Geometry: final body of the model. Coordinates: model frame, mm. A direction names the side the tool comes from. Give positions to 0.01 mm unless a question says otherwise; leave off trailing zeros. Write each loop counter-clockwise with the first axis right and the second up, starting at its lowest first coordinate (ties: lowest second). Pieces come first, ordered by that corner, then holes.
Q1. Cut plane A-A on z = -7. Count the separate pieces of the cut face and the enclosed holes in it, plus the area to 3 significant figures.
Q2. Cut plane B-B on x = 120.5. Return the cut outline in (y, z), plus the area to 3 significant figures.
Q3. Line query: L1, parallel to Y at x = 165.5, z = 2.5; L2, parallel to X at y = -71, z = 0.25; L3, parallel to Y at x = 109.5, z = -10. Output: solid intervals per line, ascending.
Q4. Reachability of faces 5 (the face through (84.883, -60.532, 0.128)), 6 (the face through (111.171, -67.236, -6.949)) from +Z, -Z, +X, -X, +Y, -Y: full face, straight path, thin tool, end or side. Return the list, or none.
Q5. Cut plane D-D on y = -62. Return the cut outline in (x, z).
Q6. Draft query along X for faces 1 (the face through (131, -60.25, 1)), 2 (the face through (121, -99, 12.6)), 3 (the face through (179.11, -97.97, 0.13)), 4 (the face through (82.898, -79, 0)). Return one class per face: pulls with the +X half, pulls with the -X half, needs draft (parallel to the pull), parting line crosses it, or undercut.
Q7. Cut plane C-C on z = 6.75. Return the cut outline in (x, y).
Q8. Pin query (flat end, axial travel): pin 1 (4.5 mm diameter, centred on x = 111, y = -67, fed in from +Z); pin 2 (1.7 mm diameter, centred on x = 173.5, y = -92.49, fed in from +Z); pin 3 (1.5 mm diameter, centred on y = -94.5, z = -0.5, fed in from -X). Return the tip coordinate at first contact, or that it passes through.
```python
from build123d import *

# Parameters (mm, degrees)
SKETCH002_R      = 2.7
SKETCH002_R_2    = 1.4
EXTRUDE001_DEPTH = 7
EXTRUDE002_DEPTH = 23
EXTRUDE_DEPTH    = 1.6


with BuildPart() as obj1:
    # Sketch002 (on Face10 of Extrude) → Extrude001 (new body)
    with BuildSketch(Plane.XY.offset(-10.4)):
        with Locations((90.524621, -65.993824)):
            Circle(SKETCH002_R)
        with Locations((90.524621, -65.993824)):
            Circle(SKETCH002_R_2, mode=Mode.SUBTRACT)
        with Locations((90.502441, -92.471822)):
            Circle(SKETCH002_R)
        with Locations((90.502441, -92.471822)):
            Circle(SKETCH002_R_2, mode=Mode.SUBTRACT)
        with Locations((153.513474, -66.00515)):
            Circle(SKETCH002_R)
        with Locations((153.513474, -66.00515)):
            Circle(SKETCH002_R_2, mode=Mode.SUBTRACT)
        with Locations((153.502167, -92.48777)):
            Circle(SKETCH002_R)
        with Locations((153.502167, -92.48777)):
            Circle(SKETCH002_R_2, mode=Mode.SUBTRACT)
    extrude(amount=EXTRUDE001_DEPTH)


with BuildPart() as obj1_1:
    # Extrude001 placement: moved
    add(obj1.part.moved(Location((20, 0, 0))))


with BuildPart() as walls:
    # Sketch → Extrude002 (new body)
    with BuildSketch(Plane.XY):
        with BuildLine():
            Line((89.498192, -99.850084), (174.498192, -99.850084))
            ThreePointArc((174.498192, -99.850084), (179.165097, -97.916989), (181.098192, -93.250084))
            Line((181.098192, -93.250084), (181.098192, -65.250084))
            ThreePointArc((181.098192, -65.250084), (179.165097, -60.583179), (174.498192, -58.650084))
            Line((174.498192, -58.650084), (89.498192, -58.650084))
            ThreePointArc((89.498192, -58.650084), (84.831287, -60.583179), (82.898192, -65.250084))
            Line((82.898192, -65.250084), (82.898192, -93.250084))
            ThreePointArc((82.898192, -93.250084), (84.831287, -97.916989), (89.498192, -99.850084))
        make_face()
        with BuildLine():
            Line((89.498192, -60.250084), (174.498192, -60.250084))
            ThreePointArc((179.498192, -65.250084), (178.033726, -61.71455), (174.498192, -60.250084))
            Line((179.498192, -65.250084), (179.498192, -93.250084))
            ThreePointArc((174.498192, -98.250084), (178.033726, -96.785618), (179.498192, -93.250084))
            Line((174.498192, -98.250084), (89.498192, -98.250084))
            ThreePointArc((84.498192, -93.250084), (85.962658, -96.785618), (89.498192, -98.250084))
            Line((84.498192, -93.250084), (84.498192, -65.250084))
            ThreePointArc((89.498192, -60.250084), (85.962658, -61.71455), (84.498192, -65.250084))
        make_face(mode=Mode.SUBTRACT)
    extrude(amount=EXTRUDE002_DEPTH)


with BuildPart() as walls_1:
    # Extrude002 placement: moved
    add(walls.part.moved(Location((0, 0, -10.4))))


with BuildPart() as doos:
    # Sketch001 → Extrude (new body)
    with BuildSketch(Plane.XY):
        with BuildLine():
            Line((89.498192, -99.850084), (174.498192, -99.850084))
            ThreePointArc((174.498192, -99.850084), (179.165097, -97.916989), (181.098192, -93.250084))
            Line((181.098192, -93.250084), (181.098192, -65.250084))
            ThreePointArc((181.098192, -65.250084), (179.165097, -60.583179), (174.498192, -58.650084))
            Line((174.498192, -58.650084), (89.498192, -58.650084))
            ThreePointArc((89.498192, -58.650084), (84.831287, -60.583179), (82.898192, -65.250084))
            Line((82.898192, -65.250084), (82.898192, -93.250084))
            ThreePointArc((82.898192, -93.250084), (84.831287, -97.916989), (89.498192, -99.850084))
        make_face()
    extrude(amount=EXTRUDE_DEPTH)


with BuildPart() as doos_1:
    # Extrude placement: moved
    add(doos.part.moved(Location((0, 0, -12))))

    # Fusion: union obj1, Walls
    add(obj1_1.part)
    add(walls_1.part)


solid = doos_1.part
```
Data:
1. separate pieces: 5
1. enclosed holes: 5
1. area: 487 mm2
2. outline: (-99.85, -12) - (-58.65, -12) - (-58.65, 12.6) - (-60.25, 12.6) - (-60.25, -10.4) - (-98.25, -10.4) - (-98.25, 12.6) - (-99.85, 12.6) - close
2. area: 140 mm2
3. L1: y = -99.85 to -98.25, -60.25 to -58.65
3. L2: x = 82.9 to 84.5, 179.5 to 181.1
3. L3: y = -99.85 to -98.25, -94.98 to -93.45, -91.49 to -89.96, -68.49 to -66.95, -65.04 to -63.5, -60.25 to -58.65
4. face 5: +Z, -Z, -X, +Y
4. face 6: +Z
5. outline: (83.75, -12) - (180.24, -12) - (180.24, 12.6) - (178.3, 12.6) - (178.3, -10.4) - (85.7, -10.4) - (85.7, 12.6) - (83.75, 12.6) - close
6. face 1: undercut
6. face 2: needs draft
6. face 3: pulls with the +X half
6. face 4: pulls with the -X half
7. outline: (82.9, -93.25) arc R6.6 ccw to (89.5, -99.85) - (174.5, -99.85) arc R6.6 ccw to (181.1, -93.25) - (181.1, -65.25) arc R6.6 ccw to (174.5, -58.65) - (89.5, -58.65) arc R6.6 ccw to (82.9, -65.25) - close; hole (84.5, -93.25) arc R5 ccw to (89.5, -98.25) - (174.5, -98.25) arc R5 ccw to (179.5, -93.25) - (179.5, -65.25) arc R5 ccw to (174.5, -60.25) - (89.5, -60.25) arc R5 ccw to (84.5, -65.25) - close
8. pin 1: stops at z = -3.4
8. pin 2: stops at z = -10.4
8. pin 3: stops at x = 82.92
